from build123d import *

# Parameters (mm, degrees)
SKETCH1_W                                     = 19.05
SKETCH1_H                                     = 19.05
BOSS_EXTRUDE1_DEPTH                           = 19.05
TAPPED_HOLE_FOR_10_24_HELICOIL1_D             = 5.15874
CSK_FOR_6_FLAT_HEAD_MACHINE_SCREW1_AT_2_COUNT = 2
CSK_FOR_6_FLAT_HEAD_MACHINE_SCREW1_AT_2_PITCH = 7.9375
CSK_FOR_6_FLAT_HEAD_MACHINE_SCREW1_AT_3_COUNT = 2
CSK_FOR_6_FLAT_HEAD_MACHINE_SCREW1_AT_3_PITCH = 13.915775446
CSK_FOR_6_FLAT_HEAD_MACHINE_SCREW1_AT_4_COUNT = 2
CSK_FOR_6_FLAT_HEAD_MACHINE_SCREW1_AT_4_PITCH = 11.43
CHAMFER2_SIZE                                 = 5.08


with BuildPart() as part:
    # Sketch1 → Boss-Extrude1 (new body)
    with BuildSketch(Plane(origin=(0, 0, 0), x_dir=(1, 0, 0), z_dir=(0, 1, 0))):
        Rectangle(SKETCH1_W, SKETCH1_H)
    extrude(amount=BOSS_EXTRUDE1_DEPTH)

    # Tapped Hole for #10-24 Helicoil1 (through all)
    with Locations(Plane.XZ):
        with Locations((0, 0)):
            Hole(TAPPED_HOLE_FOR_10_24_HELICOIL1_D / 2)

    # Sketch5 → CSK for #6 Flat Head Machine Screw1 (revolve, cut)
    with BuildSketch(Plane(origin=(-9.525, 5.55625, 5.715), x_dir=(0, 0, 1), z_dir=(0, 1, 0))):
        Polygon((0, 0), (0, 19.05), (2.15265, 19.05), (2.15265, 6.679759826), (3.5433, 5.08), (3.5433, 0), align=None)
    csk_for_6_flat_head_machine_screw1 = revolve(axis=Axis((-15.875, 5.55625, 5.715), (1, 0, 0)), mode=Mode.SUBTRACT)

    # CSK for #6 Flat Head Machine Screw1 at 2: CSK for #6 Flat Head Machine Screw1 ×2
    with Locations(*[(0, i * CSK_FOR_6_FLAT_HEAD_MACHINE_SCREW1_AT_2_PITCH, 0) for i in range(1, CSK_FOR_6_FLAT_HEAD_MACHINE_SCREW1_AT_2_COUNT)]):
        add(csk_for_6_flat_head_machine_screw1, mode=Mode.SUBTRACT)

    # CSK for #6 Flat Head Machine Screw1 at 3: CSK for #6 Flat Head Machine Screw1 ×2
    with Locations(*[Vector(0, 0.5703958094953442, -0.8213699656732957) * (i * CSK_FOR_6_FLAT_HEAD_MACHINE_SCREW1_AT_3_PITCH) for i in range(1, CSK_FOR_6_FLAT_HEAD_MACHINE_SCREW1_AT_3_COUNT)]):
        add(csk_for_6_flat_head_machine_screw1, mode=Mode.SUBTRACT)

    # CSK for #6 Flat Head Machine Screw1 at 4: CSK for #6 Flat Head Machine Screw1 ×2
    with Locations(*[(0, 0, -i * CSK_FOR_6_FLAT_HEAD_MACHINE_SCREW1_AT_4_PITCH) for i in range(1, CSK_FOR_6_FLAT_HEAD_MACHINE_SCREW1_AT_4_COUNT)]):
        add(csk_for_6_flat_head_machine_screw1, mode=Mode.SUBTRACT)

    # Chamfer2
    # the kernel refuses this chamfer: 5.08 mm, written as the material it takes off along each edge
    with BuildSketch(Plane(origin=(-9.525, -13.064149579, -9.525), x_dir=(0.9996219169112966, 0, -0.02749587661058626), z_dir=(0, 1, 0)), Plane(origin=(-9.525, -13.064149579, 9.525), x_dir=(-0.02749587661058626, 0, -0.9996219169112968), z_dir=(0, 1, 0))) as chamfer2_piece_1:
        Polygon((CHAMFER2_SIZE * 0.999621916911, -CHAMFER2_SIZE * 0.0274958766106), (-CHAMFER2_SIZE * 0.0274958766106, -CHAMFER2_SIZE * 0.999621916911), (0, 0), align=None)
    extrude(amount=45.178299158, mode=Mode.SUBTRACT)


solid = part.part
Input: part model. Units: mm. Frame: model coordinates. A direction names the side the tool comes from. Round coordinates to 2 decimals unless told otherwise and drop trailing zeros. Write each loop counter-clockwise with the first axis right and the second up, starting at its lowest first coordinate (ties: lowest second). Pieces come first, ordered by that corner, then holes.
1) Cut plane B-B (z = 0). Return the cut outline in (x, y) (3 decimals).
2) Cut plane C-C (y = 17.5). Return the cut outline in (x, z) (3 decimals).
3) Contact query for flat-ended pins moving along their axis: P1, Ø4, axis at x = -5, y = 6, coming from the +Z side (3 decimals); P2, Ø1, axis at x = -5.5, y = 10, coming from the +Z side; P3, Ø5, axis at y = 13.49, z = 5.72, coming from the -X side. Output: stop coordinate, or through.
4) Reachability of faces 5 (the cylindrical face through (3.25, 6.87, 4.01)), 6 (the cylindrical face through (-6.456, 4.492, -2.335)) from +Z, -Z, +X, -X, +Y, -Y: full face, straight path, thin tool, end or side. Return the list, or none.
5) Draft query along Z for faces 1 (the flat face through (2, 19.05, -2)), 2 (the cylindrical face through (-6.456, 13.338, 2.175)), 3 (the cylindrical face through (-6.456, 5.4, 2.175)), 4 (the flat face through (-6.38, 9.39, -7.59)). Return one class per face: pulls with the +Z half, pulls with the -Z half, needs draft (parallel to the pull), parting line crosses it, or undercut.
6) Cut plane D-D (x = 1.75). Return the cut outline in (y, z) (3 decimals).
7) Ray query, L1, parallel to Z at x = -4.75, y = 15; L2, parallel to Y at x = 1.75, z = -4.5; L3, parallel to Y at x = -2.75, z = -6.25. Return the intervals inside material, ascending.
8) Cut plane A-A (x = -2). Return the cut outline in (y, z) (3 decimals).
Geometry says:
1. outline: (-9.525, 0) - (-2.579, 0) - (-2.579, 19.05) - (-9.525, 19.05) - close; (2.579, 0) - (9.525, 0) - (9.525, 19.05) - (2.579, 19.05) - close
2. outline: (-9.525, -4.445) - (-4.445, -9.525) - (9.525, -9.525) - (9.525, 9.525) - (-4.445, 9.525) - (-9.525, 4.445) - close; hole circle Ø5.159 at (0, 0)
3. P1: stops at z = 9.525
3. P2: stops at z = 8.97
3. P3: stops at x = -3.25
4. face 5: +X, -X
4. face 6: -X
5. face 1: needs draft
5. face 2: undercut
5. face 3: undercut
5. face 4: pulls with the -Z half
6. outline: (0, -9.525) - (19.05, -9.525) - (19.05, -1.895) - (0, -1.895) - close; (0, 1.895) - (19.05, 1.895) - (19.05, 9.525) - (0, 9.525) - close; hole circle Ø4.305 at (5.556, -5.715); hole circle Ø4.305 at (5.556, 5.715); hole circle Ø4.305 at (13.494, -5.715); hole circle Ø4.305 at (13.494, 5.715)
7. L1: z = -9.22 to -8.92, -2.51 to 2.51, 8.92 to 9.22
7. L2: y = 0 to 3.78, 7.33 to 11.72, 15.27 to 19.05
7. L3: y = 0 to 3.47, 7.64 to 11.41, 15.58 to 19.05
8. outline: (0, -9.525) - (19.05, -9.525) - (19.05, -1.629) - (0, -1.629) - close; (0, 1.629) - (19.05, 1.629) - (19.05, 9.525) - (0, 9.525) - close; hole circle Ø4.305 at (5.556, -5.715); hole circle Ø4.305 at (5.556, 5.715); hole circle Ø4.305 at (13.494, -5.715); hole circle Ø4.305 at (13.494, 5.715)
